from build123d import *
from build123d.topology import SkipClean

# Parameters (mm, degrees)
BOSS_EXTRUDE1_DEPTH = 640
SKETCH22_R          = 6
CUT_EXTRUDE4_DEPTH  = 10
BOSS_EXTRUDE2_DEPTH = 63
BOSS_EXTRUDE3_DEPTH = 7
SKETCH26_R          = 6
CUT_EXTRUDE5_DEPTH  = 7
FILLET1_R           = 10
FILLET2_R           = 10


with BuildPart() as part:
    # Sketch1 → Boss-Extrude1 (new body)
    with BuildSketch(Plane.XY):
        Polygon((0, 0), (0, 70), (70, 70), (70, 63), (7, 63), (7, 0), align=None)
    extrude(amount=BOSS_EXTRUDE1_DEPTH)

    # Sketch22 → Cut-Extrude4 (cut)
    with BuildSketch(Plane(origin=(0, 70, 0), x_dir=(1, 0, 0), z_dir=(0, 1, 0))):
        with Locations((35, 0)):
            Circle(SKETCH22_R)
        with Locations((35, 500)):
            Circle(SKETCH22_R)
        with Locations(Location((35, -500, 0), (0, 0, 270))):
            Circle(SKETCH22_R)
    extrude(amount=-CUT_EXTRUDE4_DEPTH, mode=Mode.SUBTRACT)

    # Sketch23 → Boss-Extrude2 (add)
    with BuildSketch(Plane(origin=(0, 0, 0), x_dir=(1, 0, 0), z_dir=(0, 1, 0))):
        Polygon((0, -640), (42.5, -713.612159322), (48.562177826, -710.112159322), (7, -640), align=None)
    extrude(amount=BOSS_EXTRUDE2_DEPTH)

    # Sketch25 → Boss-Extrude3 (add)
    with BuildSketch(Plane(origin=(0, 63, 0), x_dir=(1, 0, 0), z_dir=(0, 1, 0))):
        Polygon((70, -640), (0, -640), (42.5, -713.612159322), (70, -713.612159322), align=None)
    extrude(amount=BOSS_EXTRUDE3_DEPTH)

    # Sketch26 → Cut-Extrude5 (cut)
    with BuildSketch(Plane(origin=(-275.556719825, 0, 163.348804279), x_dir=(-0.5099316128113042, 0, -0.8602149442178172), z_dir=(0.8602149442178172, 0, -0.5099316128113042))):
        with Locations((-614.36248118, 31.5)):
            Circle(SKETCH26_R)
        with Locations((-575.367085589, 31.5)):
            Circle(SKETCH26_R)
    extrude(amount=-CUT_EXTRUDE5_DEPTH, mode=Mode.SUBTRACT)

    # Mirror1: part across plane


with BuildPart() as part_1:
    with SkipClean():  # the faces are left unmerged after this step: merging them gives an invalid solid
        add(part.part)
        add(part.part.mirror(Plane.XY))

    # Fillet1
    fillet1_edges = [part_1.edges().sort_by_distance(p)[0] for p in [
        (0, 35, 640),
        (0, 35, -640),
    ]]
    fillet(fillet1_edges, radius=FILLET1_R)

    # Fillet2
    fillet2_edges = [part_1.edges().sort_by_distance(p)[0] for p in [
        (7, 31.5, -640),
        (7, 31.5, 640),
    ]]
    fillet(fillet2_edges, radius=FILLET2_R)


solid = part_1.part
Geometry check sheet. Reference: the model listing, model coordinates, mm. A direction names the side the tool comes from. Coordinates: 2 decimals unless noted, no trailing zeros. Order: outer loops, then holes, each group sorted by start corner. A loop starts at its lowest first (then second) coordinate and runs counter-clockwise, first axis right, second up. Notation, with made-up numbers: M -19,65 L 4,65 A26 ccw 4,88 Z; hole C 71,-10.75 d10. An arc over 180 degrees is marked long. Use CSV: the item, a comma, the result in double quotes.
Item 1: Tool access check on faces 4 (the flat face through (38, 63, 10)), 5 (the flat face through (6, 0, 3)). Record the directions out of +Z, -Z, +X, -X, +Y, -Y that give a thin tool (end or side, any length) a straight path to the whole face; none if there is none.
Returned:
face 4,"+X, -Y"
face 5,"+Z, -Z, +X, -X, -Y"
Item 2: Thickness scan on line 1 along X through (y, z) = (64.75, -500); line 2 along Y through (x, z) = (12, -37); line 3 along X through (y, z) = (19, 397). Record the ranges inside material, lowest first.
Returned:
line 1,"x = 0 to 29, 41 to 70"
line 2,"y = 63 to 70"
line 3,"x = 0 to 7"
Item 3: Gauge pin test, flat ends, axial feed: pin 1 Ø12 at (x, z) = (57, 33.5) entering from -Y; pin 2 Ø12 at (y, z) = (35.5, 258) entering from +X. Record the tip position at first contact, or that the pin passes through.
Returned:
pin 1,"stops at y = 63"
pin 2,"stops at x = 7"
Item 4: Mould release check, pull along Z, two halves, no side actions. Record for faces 1 (the flat face through (7, 32, 9)), 2 (the flat face through (21.632, 34.51, 677.467)), 3 (the flat face through (0, 35, 9)): pulls with the +Z half, pulls with the -Z half, needs draft (parallel to the pull), parting line crosses it, or undercut.
Returned:
face 1,"undercut"
face 2,"pulls with the +Z half"
face 3,"needs draft"
Item 5: Cross-section at A-A on z = -362. Record the cut outline in (x, y).
Returned:
outline,"M 0,0 L 7,0 L 7,63 L 70,63 L 70,70 L 0,70 Z"
